Geometry check sheet. Reference: the model listing, model coordinates, mm. Face numbers are marked on the shaded views. A direction names the side the tool comes from. Round coordinates to 2 decimals unless told otherwise and drop trailing zeros. Order: outer loops, then holes, each group sorted by start corner. A loop starts at its lowest first (then second) coordinate and runs counter-clockwise, first axis right, second up. Notation, with made-up numbers: M 50.5,-22 L 82.5,-22 A33 cw 82.5,8 Z; hole C 86,-4 d1. An arc over 180 degrees is marked long. Return JSON: item names as keys, results as strings. Group by question number.
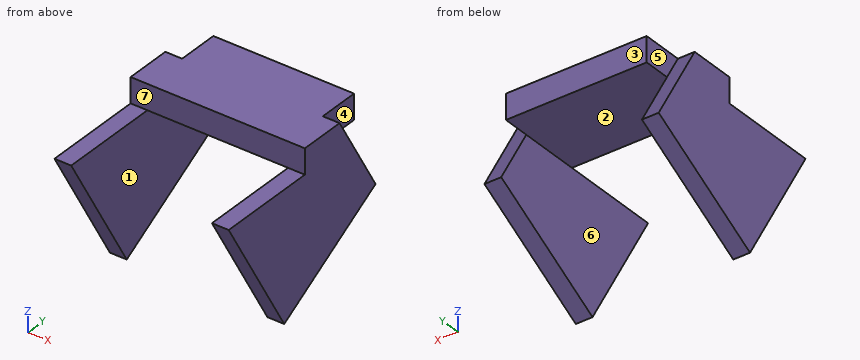
Autodesk Inventor part; units mm, degrees
ref_plane "YZ Plane" through (0, 0, 0) normal (1, 0, 0) x (0, 1, 0)
ref_plane "XZ Plane" through (0, 0, 0) normal (0, 1, 0) x (-1, 0, 0)
ref_plane "XY Plane" through (0, 0, 0) normal (0, 0, 1) x (1, 0, 0)
ref_plane "Work Plane1" through (0, 0, 0) normal (0, 0, 1) x (1, 0, 0)
sketch "Sketch1" plane through (0, 0, 0) normal (0, 0, 1) x (1, 0, 0)
  line L0 (4, -5.5111) -> (4, 5.5111) construction
  line L1 (4, 5.5111) -> (-4, 5.5111) construction
  line L2 (-4, 5.5111) -> (-4, -5.5111) construction
  line L3 (-4, -5.5111) -> (4, -5.5111) construction
  line L4 (-4, 5.5111) -> (4.1522, 5.5111) construction
  line L5 (4.1522, 5.5111) -> (4.1522, 0.5111) construction
  line L6 (4.1522, 0.5111) -> (-4, 0.5111) construction
  line L7 (-4, 0.5111) -> (-4, 5.5111) construction
  line L8 (-4.12, 0.3911) -> (4.2722, 0.3911)
  line L9 (4.2722, 0.3911) -> (4.2722, 5.6311)
  line L10 (4.2722, 5.6311) -> (-4.12, 5.6311)
  line L11 (-4.12, 5.6311) -> (-4.12, 0.3911)
  point P0 (0, 0)
  dimension "d0" = 5
  dimension "d1" = 0.12
extrude "Extrusion1" add sketch "Sketch1" along normal blind 1.5
sketch "Sketch2" plane through (4.2722, 0.3911, 0) normal (1, 0, 0) x (0, 0, -1)
  line L0 (-1.5, 0) -> (-1.5, 5.24) construction
  line L1 (4.4205, 6.1762) -> (4.9103, 6.459) construction
  line L2 (4.9103, 6.459) -> (2.5, 10.6336) construction
  line L3 (2.5, 10.6336) -> (0.5, 9.4789) construction
  line L4 (0.5, 9.4789) -> (0.5, 5.12) construction
  line L5 (0.5, 5.12) -> (0, 5.12) construction
  line L6 (0, -5.9023) -> (0, 5.12) construction
  line L7 (0.5, -5.9023) -> (0, -5.9023) construction
  line L8 (8.6705, -1.185) -> (0.5, -5.9023) construction
  line L9 (8.6705, -1.185) -> (4.4205, 6.1762) construction
  line L10 (0.4678, -5.7823) -> (0.12, -5.7823) construction
  line L11 (0.12, -5.7823) -> (0.12, 5) construction
  line L12 (0.12, 5) -> (0.62, 5) construction
  line L13 (0.62, 5) -> (0.62, 9.4097) construction
  line L14 (0.62, 9.4097) -> (2.4561, 10.4697) construction
  line L15 (2.4561, 10.4697) -> (4.7463, 6.5029) construction
  line L16 (4.7463, 6.5029) -> (4.2566, 6.2201) construction
  line L17 (4.2566, 6.2201) -> (8.5066, -1.1411) construction
  line L18 (8.5066, -1.1411) -> (0.4678, -5.7823) construction
  line L19 (6.2093, 7.209) -> (-21.3823, -8.721) construction
  line L20 (4.3166, 6.1162) -> (-1.5, 2.758)
  line L21 (-1.5, 2.758) -> (-1.5, 0)
  line L22 (-1.5, 0) -> (0.12, 0)
  line L23 (8.5066, -1.1411) -> (0, -6.0524)
  line L24 (0, -6.0524) -> (0, 0)
  line L25 (8.5066, -1.1411) -> (4.3166, 6.1162)
  line L26 (3.4506, 5.6162) -> (7.6406, -1.6411)
  line L27 (0, -6.0524) -> (0, 0)
  line L28 (0, 0) -> (-1.5, 0)
  point P0 (0, -0.3911)
  dimension "d4" = 0.12
  dimension "d5" = 1
extrude "Extrusion2" add sketch "Sketch2" along normal blind 1 contours L26 L23 L24 L22 L21 L20
ref_plane "Work Plane2" through (0.0761, 5.6311, 1.5) normal (1, 0, 0) x (0, 0, -1)
mirror "Mirror1" about plane through (0.0761, 5.6311, 1.5) normal (1, 0, 0) of "Extrusion2"
properties part number "PTFEFilter_clamp"
Q1. Release check for a two-part mould opening along X. For the marked faces 1, 2, 3 and 4 record: +X half, -X half, draft (parallel to the pull), parting line (faces both ways), or undercut.
Q2. Set-up check for the marked faces 5, 6 and 7: record each of +Z, -Z, +X, -X, +Y, -Y from which the full face is reachable in a straight line by a thin tool's end or side.
Q3. Section check B-B on z = -5. Record the cut outline in (x, y), plus the area to 3 significant figures.
Q4. Section check A-A on y = 4.25. Record the cut outline in (x, z).
Q5. Depth check by flat-ended pin: pin 1 Ø2 at (x, y) = (-2.5, -4.5) entering from +Z; pin 2 Ø5 at (x, y) = (-4, -2.5) entering from +Z; pin 3 Ø4 at (x, y) = (-0.5, 2.5) entering from -Z; pin 4 Ø1.2 at (y, z) = (5, 0.5) entering from +X. Enter the tip coordinate at first touch or a pass-through.
Q6. Material ranges on line 1 along X through (y, z) = (-4, -2.75); line 2 along Z through (x, y) = (0.75, 2.5); line 3 along Z through (x, y) = (4.5, -3), recorded low to high.
Q7. Section check D-D on y = 1.25. Record the cut outline in (x, z), plus the area to 3 significant figures.
Q8. Section check C-C on y = -1. Record the cut outline in (x, z), plus the area to 3 significant figures.
Geometry check:
{
 "1": {"face 1": "undercut", "face 2": "undercut", "face 3": "draft", "face 4": "+X half"},
 "2": {"face 5": "+Z, -X, +Y", "face 6": "-Z, +Y, -Y", "face 7": "+Z, +X, -X, -Y"},
 "3": {"outline": "M -5.12,-2.77 L -4.12,-2.77 L -4.12,3.32 L -5.12,3.32 Z; M 4.27,-2.77 L 5.27,-2.77 L 5.27,3.32 L 4.27,3.32 Z", "area": "12.2 mm^2"},
 "4": {"outline": "M -5.12,-4.47 L -4.12,-4.47 L -4.12,-0.41 L -5.12,-0.41 Z; M -4.12,0 L 4.27,0 L 4.27,1.5 L -4.12,1.5 Z; M 4.27,-4.47 L 5.27,-4.47 L 5.27,-0.41 L 4.27,-0.41 Z"},
 "5": {"pin 1": "passes through", "pin 2": "stops at z = 0", "pin 3": "stops at z = 0", "pin 4": "stops at x = 4.27"},
 "6": {"line 1": "x = -5.12 to -4.12, 4.27 to 5.27", "line 2": "z = 0 to 1.5", "line 3": "z = -4.61 to 0"},
 "7": {"outline": "M -5.12,-6.2 L -4.12,-6.2 L -4.12,0 L 4.27,0 L 4.27,-6.2 L 5.27,-6.2 L 5.27,1.5 L -5.12,1.5 Z", "area": "28.0 mm^2"},
 "8": {"outline": "M -5.12,-7.5 L -4.12,-7.5 L -4.12,0 L -5.12,0 Z; M 4.27,-7.5 L 5.27,-7.5 L 5.27,0 L 4.27,0 Z", "area": "15.0 mm^2"}
}
